Could you check a few things on this drawing? It's one solid part, dimensions in mm from its lowest x, y, z. Coordinates: 2 decimals unless noted, no trailing zeros. Write each loop counter-clockwise with the first axis right and the second up, starting at its lowest first coordinate (ties: lowest second). Pieces come first, ordered by that corner, then holes.
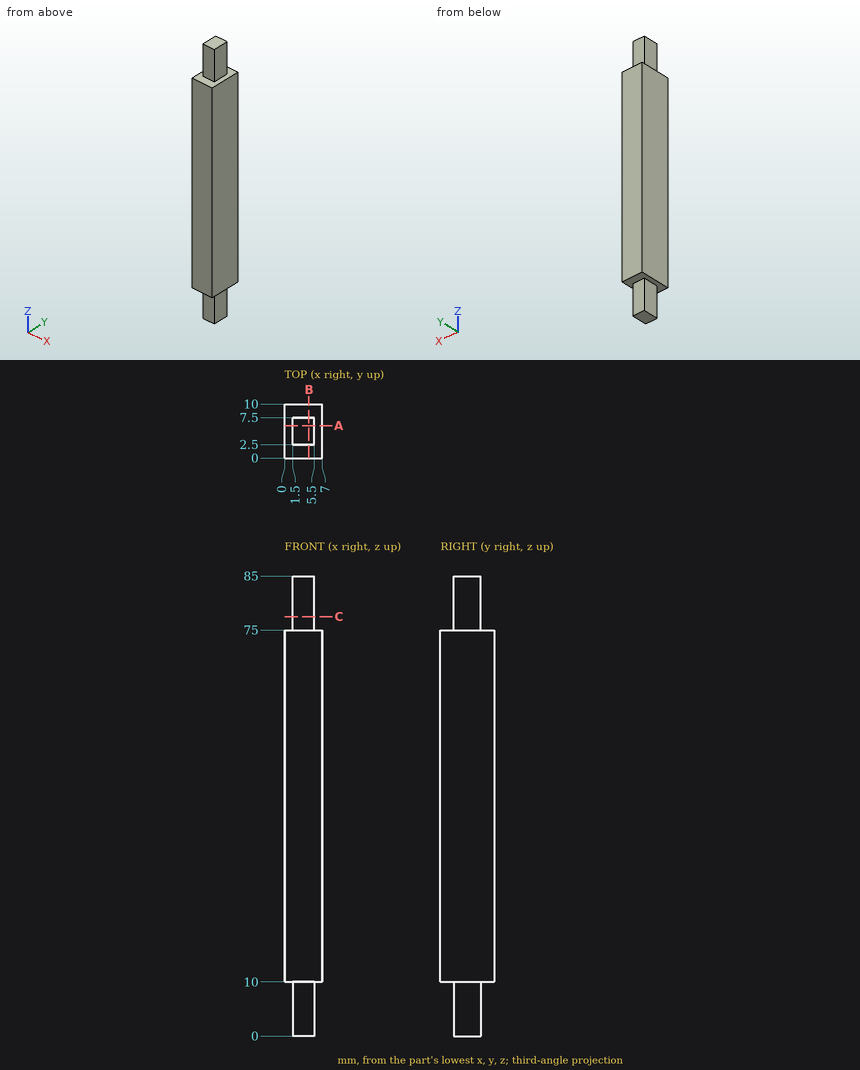
1) Imagine slicing it at C-C on z = 77.5. Please give me the cut outline in (x, y), then the cut area to 3 significant figures.
Values follow:
outline: (1.5, 2.5) - (5.5, 2.5) - (5.5, 7.5) - (1.5, 7.5) - close
area: 20.0 mm2
2) Imagine slicing it at B-B on x = 4.5. Please give me the cut outline in (y, z), then the cut area to 3 significant figures.
Values follow:
outline: (0, 10) - (2.5, 10) - (2.5, 0) - (7.5, 0) - (7.5, 10) - (10, 10) - (10, 75) - (7.5, 75) - (7.5, 85) - (2.5, 85) - (2.5, 75) - (0, 75) - close
area: 750 mm2
3) Imagine slicing it at A-A on y = 6. Please give me the cut outline in (x, z), then the cut area to 3 significant figures.
Values follow:
outline: (0, 10) - (1.5, 10) - (1.5, 0) - (5.5, 0) - (5.5, 10) - (7, 10) - (7, 75) - (5.5, 75) - (5.5, 85) - (1.5, 85) - (1.5, 75) - (0, 75) - close
area: 535 mm2
4) Will these pins go through, and if not, where does the flat tip stop? pin 1 (2.5 mm diameter, centred on y = 4, z = 81, fed in from +X); pin 2 (1.2 mm diameter, centred on x = 3.5, z = 78, fed in from -Y); pin 3 (4 mm diameter, centred on y = 4, z = 80, fed in from -X).
Values follow:
pin 1: stops at x = 5.5
pin 2: stops at y = 2.5
pin 3: stops at x = 1.5
5) I need wall thicknesses on probe 1 along Z at (x, y) = (4.5, 2); probe 2 along Y at (x, z) = (2.25, 6.5); probe 3 along X at (y, z) = (6.25, 7). Which ranges of each line are inside material? Lowest first, please.
Values follow:
probe 1: z = 10 to 75
probe 2: y = 2.5 to 7.5
probe 3: x = 1.5 to 5.5
